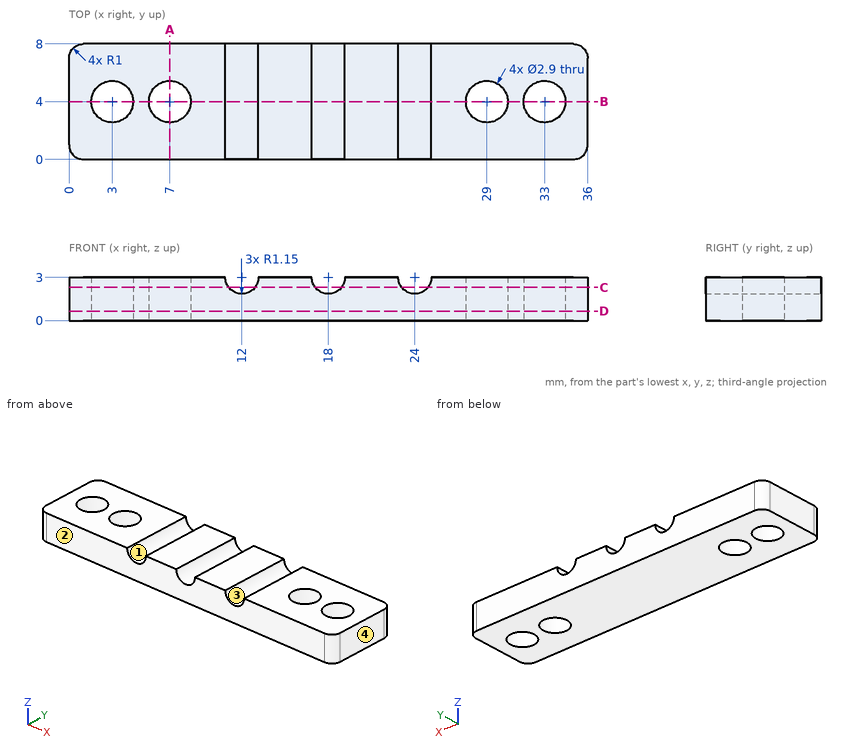
Design review of the part shown in the three views and the two pictorial views. Dimensions are in mm from the part's minimum x, y and z. Round coordinates to 2 decimals unless told otherwise and drop trailing zeros. Loops run counter-clockwise (first coordinate to the right, second up) from the corner with the lowest first, then second, coordinate; pieces in that order, holes last.
Q1. Add section D-D on z = 0.65. Write out the cut boundary in (x, y), plus the area to 3 significant figures.
Result sheet:
outline: (0, 1) arc R1 ccw to (1, 0) - (35, 0) arc R1 ccw to (36, 1) - (36, 7) arc R1 ccw to (35, 8) - (1, 8) arc R1 ccw to (0, 7) - close; hole circle Ø2.9 at (3, 4); hole circle Ø2.9 at (7, 4); hole circle Ø2.9 at (29, 4); hole circle Ø2.9 at (33, 4)
area: 261 mm2
Q2. Add section A-A on x = 7. Write out the cut boundary in (y, z).
Result sheet:
outline: (0, 0) - (2.55, 0) - (2.55, 3) - (0, 3) - close; (5.45, 0) - (8, 0) - (8, 3) - (5.45, 3) - close
Q3. To check wall thickness, follow line 1 along Y through (x, z) = (33, 2); line 2 along X through (y, z) = (4.75, 0.6); line 3 along X through (y, z) = (6.25, 2.8). State the ranges of each line that lie inside material, in increasing order.
Result sheet:
line 1: y = 0 to 2.55, 5.45 to 8
line 2: x = 0 to 1.76, 4.24 to 5.76, 8.24 to 27.76, 30.24 to 31.76, 34.24 to 36
line 3: x = 0 to 10.87, 13.13 to 16.87, 19.13 to 22.87, 25.13 to 36
Q4. Insertion check: pin 1 Ø1.5 at (x, z) = (10, 0.5) entering from -Y. The pin has a flat end and moves straight along its axis. Give the tip position at first contact, or say it passes through.
Result sheet:
pin 1: stops at y = 0
Q5. Add section B-B on y = 4. Write out the cut boundary in (x, z), plus the area to 3 significant figures.
Result sheet:
outline: (0, 0) - (1.55, 0) - (1.55, 3) - (0, 3) - close; (4.45, 0) - (5.55, 0) - (5.55, 3) - (4.45, 3) - close; (8.45, 0) - (27.55, 0) - (27.55, 3) - (25.15, 3) arc R1.15 cw to (22.85, 3) - (19.15, 3) arc R1.15 cw to (16.85, 3) - (13.15, 3) arc R1.15 cw to (10.85, 3) - (8.45, 3) - close; (30.45, 0) - (31.55, 0) - (31.55, 3) - (30.45, 3) - close; (34.45, 0) - (36, 0) - (36, 3) - (34.45, 3) - close
area: 67.0 mm2
Q6. Add section C-C on z = 2.3. Write out the cut boundary in (x, y).
Result sheet:
outline: (0, 1) arc R1 ccw to (1, 0) - (11.09, 0) - (11.09, 8) - (1, 8) arc R1 ccw to (0, 7) - close; (12.91, 0) - (17.09, 0) - (17.09, 8) - (12.91, 8) - close; (18.91, 0) - (23.09, 0) - (23.09, 8) - (18.91, 8) - close; (24.91, 0) - (35, 0) arc R1 ccw to (36, 1) - (36, 7) arc R1 ccw to (35, 8) - (24.91, 8) - close; hole circle Ø2.9 at (3, 4); hole circle Ø2.9 at (7, 4); hole circle Ø2.9 at (29, 4); hole circle Ø2.9 at (33, 4)
Q7. Mouldability with a two-part tool opening along X and no side actions: class the marked faces 1, 2, 3 and 4 as +X half, -X half, draft (parallel to the pull), parting line (faces both ways), or undercut.
Result sheet:
face 1: undercut
face 2: draft
face 3: undercut
face 4: +X half
